from build123d import *

# Parameters (mm, degrees)
F1_DEPTH = 25.4
F2_W     = 58.1890912727
F2_H     = 43.6418224126
F3_DEPTH = 25.4
F4_R     = 5.08


with BuildPart() as f1:
    # F0 (on Front) → F1 (new body)
    with BuildSketch(Plane.XZ):
        Polygon((-36.4606332477, -31.5460583245), (20.3657772835, 62.8072192942), (-89.7597633302, 64.8436956108), align=None)
    extrude(amount=F1_DEPTH)

    # F2 (on Front) + F1_face (on face) → F3 (join)
    with BuildSketch(Plane.XZ):
        with Locations((-34.9458768032, 41.4752056822)):
            Rectangle(F2_W, F2_H)
    with BuildSketch(Plane(origin=(-35.2848730981, -25.4, 32.0349521935), x_dir=(1, 0, 0), z_dir=(0, -1, 0))):
        Polygon((-1.1757601496, -63.581010518), (55.6506503816, 30.7722671007), (-54.4748902321, 32.8087434173), align=None)
    extrude(amount=-F3_DEPTH)

    # F4
    f4_edges = [f1.edges().sort_by_distance(p)[0] for p in [
        (-8.047428, -25.4, 15.63058),
        (-34.696993, -25.4, 63.825457),
        (-63.110198, -25.4, 16.648819),
    ]]
    fillet(f4_edges, radius=F4_R)


solid = f1.part
For this review, take the finished solid that the model builds, in its own axes (mm). A direction names the side the tool comes from. Give positions to 0.01 mm unless a question says otherwise; leave off trailing zeros. Order: outer loops, then holes, each group sorted by start corner. A loop starts at its lowest first (then second) coordinate and runs counter-clockwise, first axis right, second up. Notation, with made-up numbers: (60.25, 51) -> (107.25, 51) arc R26 ccw to (107.25, 77) -> close; hole circle Ø9 at (-37.5, -30). An arc over 180 degrees is marked (long way). Write item = value, one per line.
1) Insertion check: pin 1 (4 mm diameter, centred on x = -14.5, y = -10.5, fed in from +Z); pin 2 (12 mm diameter, centred on x = -63.5, y = 10, fed in from +Z); pin 3 (1 mm diameter, centred on x = -54.5, y = -8.5, fed in from +Z). Each pin has a flat end and moves straight along its axis. Give the tip position at first contact, or say it passes through.
Findings:
pin_1 = 63.49
pin_2 = 63.3
pin_3 = 64.2
2) We need section B-B, the plane y = 19.5. Give the boundary of the cut face in (x, z).
Findings:
outline = (-64.04, 19.65) -> (-5.85, 19.65) -> (-5.85, 63.3) -> (-64.04, 63.3) -> close
3) We need section A-A, the plane y = -11. Give the boundary of the cut face in (x, z), and give its area (3 significant figures).
Findings:
outline = (-89.76, 64.84) -> (-36.46, -31.55) -> (20.37, 62.81) -> close
area = 5,250 mm^2
4) To check wall thickness, follow L1, parallel to Z at x = -41.5, y = 1.5; L2, parallel to X at y = 11.5, z = 61; L3, parallel to Y at x = 7.5, z = 52. State the ranges of each line that lie inside material, in increasing order. Write a range as from..to.
Findings:
L1 = 19.65..63.3
L2 = -64.04..-5.85
L3 = -25.4..0
5) For faces 1 (the face through (-35, 13, 19.654)), 2 (the face through (-35.495, -23.872, 62.391)), 3 (the face through (-5.851, 13, 41)), list the 3-axis set-ups (+Z, -Z, +X, -X, +Y, -Y) from which the entire face can be reached by the end or side of a thin tool; tool diameter is ignored.
Findings:
face_1 = -Z, +X, -X, +Y
face_2 = +Z, +X, -Y
face_3 = +Z, -Z, +X, +Y
